Read the model definition and answer for the solid it produces. Units are mm, in the model's axes. Face numbers are marked on the shaded views. A direction names the side the tool comes from. Coordinates: 2 decimals unless noted, no trailing zeros. Write each loop counter-clockwise with the first axis right and the second up, starting at its lowest first coordinate (ties: lowest second). Pieces come first, ordered by that corner, then holes.
(1) Section C-C on z = 13 is taken. Write down the section's boundary in (x, y).
(2) Which of the six approach directions +Z, -Z, +X, -X, +Y, -Y give full straight-line access (tool end or side, diameter ignored) to the marked faces 4 and 5?
(3) Section B-B on z = 9.75 is taken. Write down the section's boundary in (x, y).
(4) Find the intervals of material crossed by probe 1 along Y at (x, z) = (0, 2.4); probe 2 along Z at (x, y) = (5.5, -8.5) (3 decimals); probe 3 along X at (y, z) = (7, 3.5), in increasing order.
(5) Given pin 1 (1 mm diameter, centred on x = 1, z = 5.5, fed in from -Y); pin 2 (8 mm diameter, centred on y = -18.5, z = 4.5, fed in from -X); pin 3 (1 mm diameter, centred on x = -6, z = 3, fed in from +Y), each flat-ended and moving along its own axis, determine where each tip first touches the part or whether it passes through.
(6) The mould has two halves that part along X. Classify the marked faces 1, 2 and 3: +X half, -X half, draft (parallel to the pull), parting line (faces both ways), or undercut.
(7) Section A-A on y = 0 is taken. Write down the section's boundary in (x, z) (1 decimal), then the cut area to 3 significant figures.
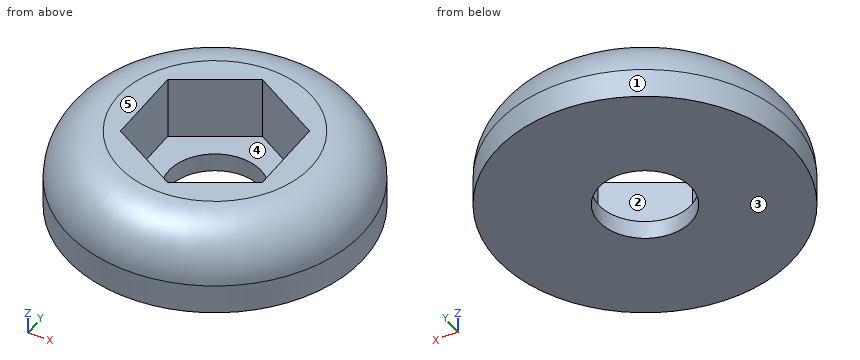
from build123d import *

# Parameters (mm, degrees)
F0_R     = 25.4
F1_DEPTH = 13.97
F0_R_2   = 7.9375
F2_DEPTH = 3.175
F3_R     = 8.89


with BuildPart() as f1:
    # F0 (on Top) → F1 (new body)
    with BuildSketch(Plane.XY):
        Circle(F0_R)
        Polygon((0, 13.956173), (12.0864, 6.978086), (12.0864, -6.978086), (0, -13.956173), (-12.0864, -6.978086), (-12.0864, 6.978086), align=None, mode=Mode.SUBTRACT)
    extrude(amount=F1_DEPTH)

    # F0 (on Top) → F2 (join)
    with BuildSketch(Plane.XY):
        Polygon((12.0864, -6.978086), (12.0864, 6.978086), (0, 13.956173), (-12.0864, 6.978086), (-12.0864, -6.978086), (0, -13.956173), align=None)
        Circle(F0_R_2, mode=Mode.SUBTRACT)
    extrude(amount=F2_DEPTH)

    # F3
    f3_edges = [f1.edges().sort_by_distance(p)[0] for p in [
        (-25.4, 0, 13.97),
    ]]
    fillet(f3_edges, radius=F3_R)


solid = f1.part
Response:
1. outline: circle Ø41.1 at (0, 0); hole (-12.09, -6.98) - (0, -13.96) - (12.09, -6.98) - (12.09, 6.98) - (0, 13.96) - (-12.09, 6.98) - close
2. face 4: +Z
2. face 5: +Z, +X, -X, +Y, -Y
3. outline: circle Ø48.15 at (0, 0); hole (-12.09, -6.98) - (0, -13.96) - (12.09, -6.98) - (12.09, 6.98) - (0, 13.96) - (-12.09, 6.98) - close
4. probe 1: y = -25.4 to -7.94, 7.94 to 25.4
4. probe 2: z = 0 to 3.175
4. probe 3: x = -24.42 to -12.05, 12.05 to 24.42
5. pin 1: stops at y = -25.39
5. pin 2: stops at x = -20.85
5. pin 3: stops at y = 24.8
6. face 1: parting line
6. face 2: undercut
6. face 3: draft
7. outline: (-25.4, 0) - (-7.9, 0) - (-7.9, 3.2) - (-12.1, 3.2) - (-12.1, 14) - (-16.5, 14) arc R8.9 ccw to (-25.4, 5.1) - close; (7.9, 0) - (25.4, 0) - (25.4, 5.1) arc R8.9 ccw to (16.5, 14) - (12.1, 14) - (12.1, 3.2) - (7.9, 3.2) - close
7. area: 364 mm2
